Here's how the part is built. I have some questions about the finished solid (model axes, mm). Face numbers are marked on the shaded views. A direction names the side the tool comes from. Round coordinates to 2 decimals unless told otherwise and drop trailing zeros. Loops run counter-clockwise (first coordinate to the right, second up) from the corner with the lowest first, then second, coordinate; pieces in that order, holes last. Notation, with made-up numbers: M 44.25,13 L 73.25,13 A22 cw 73.25,46 Z; hole C 56,0 d3. An arc over 180 degrees is marked long. Answer as CSV lines item,"result".
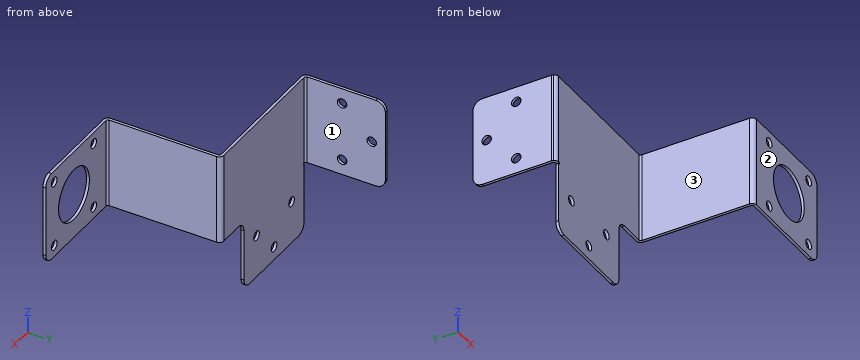
```python
from build123d import *

# Parameters (mm, degrees)
BRIDA_BASE1_DEPTH                = 1.2
BRIDA_START                      = -19
BRIDA_DE_ARISTA1_DEPTH           = 38
BRIDA_START_2                    = -19.6
BRIDA_DE_ARISTA1_2_OUTLINE_W     = 0.5366
BRIDA_DE_ARISTA1_2_OUTLINE_H     = 1.2
BRIDA_DE_ARISTA1_2_DEPTH         = 0.6
BRIDA_DE_ARISTA1_3_DEPTH         = 38
CROQUIS12_R                      = 2
CORTAR_EXTRUIR1_DEPTH            = 1.2
CROQUIS15_R                      = 2
CORTAR_EXTRUIR3_DEPTH            = 1.2
REDONDEO3_R                      = 4
BRIDA_DE_ARISTA2_STRIP_W         = 6.3732
BRIDA_DE_ARISTA2_STRIP_H         = 1.2
BRIDA_DE_ARISTA2_STRIP_CUT_DEPTH = 38
BRIDA_DE_ARISTA2_DEPTH           = 38
BRIDA_DE_ARISTA3_STRIP_W         = 6.3732
BRIDA_DE_ARISTA3_STRIP_H         = 1.2
BRIDA_DE_ARISTA3_STRIP_CUT_DEPTH = 38
BRIDA_DE_ARISTA3_DEPTH           = 38
CROQUIS22_R                      = 2
CROQUIS22_R_2                    = 11
CORTAR_EXTRUIR4_DEPTH            = 1.2
REDONDEO4_R                      = 4


# Read off the part's stored shape, not the designer's step: Brida de arista1
# Sheet-metal steps are written as plain solids
with BuildPart() as part:
    # Croquis1 → Brida base1 (new body)
    with BuildSketch(Plane(origin=(0, 0, 0), x_dir=(1, 0, 0), z_dir=(0, 1, 0))):
        Polygon((-30, -19), (30, -19), (30, 19), (15, 19), (15, 49), (-28, 49), (-28, 19), (-30, 19), align=None)
    extrude(amount=-BRIDA_BASE1_DEPTH)

    # Brida de arista1 outline → Brida de arista1 (cut)
    with BuildSketch(Plane.XY.offset(BRIDA_START)):
        with BuildLine():
            Line((-30, -1.2), (-28.0634, -1.2))
            ThreePointArc((-28.0634, -1.2), (-29.141342484, -0.872269031), (-29.854444388, 0))
            Line((-29.854444388, 0), (-30, 0))
            Line((-30, 0), (-30, -1.2))
        make_face()
    extrude(amount=BRIDA_DE_ARISTA1_DEPTH, mode=Mode.SUBTRACT)

    # Brida de arista1 2 outline → Brida de arista1 2 (cut)
    with BuildSketch(Plane.XY.offset(BRIDA_START_2)):
        with Locations((-27.7317, -0.6)):
            Rectangle(BRIDA_DE_ARISTA1_2_OUTLINE_W, BRIDA_DE_ARISTA1_2_OUTLINE_H)
    extrude(amount=BRIDA_DE_ARISTA1_2_DEPTH, mode=Mode.SUBTRACT)

    # Brida de arista1 3 outline → Brida de arista1 3 (add)
    with BuildSketch(Plane.XY.offset(BRIDA_START)):
        with BuildLine():
            Line((-29.854444388, 0), (-28.0634, 0))
            ThreePointArc((-28.0634, 0), (-28.584254855, 0.215745145), (-28.8, 0.7366))
            Line((-28.8, 0.7366), (-28.8, 33.8))
            Line((-28.8, 33.8), (-30, 33.8))
            Line((-30, 33.8), (-30, 0.7366))
            ThreePointArc((-30, 0.7366), (-29.963262642, 0.361178238), (-29.854444388, 0))
        make_face()
    extrude(amount=BRIDA_DE_ARISTA1_3_DEPTH)

    # Croquis12 → Cortar-Extruir1 (cut)
    with BuildSketch(Plane(origin=(0, 0, 0), x_dir=(1, 0, 0), z_dir=(0, 1, 0))):
        with Locations(Location((6, 30.75, 0), (0, 0, 270))):
            Circle(CROQUIS12_R)
        with Locations(Location((-19, 30.75, 0), (0, 0, 270))):
            Circle(CROQUIS12_R)
        with Locations(Location((-6.5, 43.25, 0), (0, 0, 270))):
            Circle(CROQUIS12_R)
    extrude(amount=-CORTAR_EXTRUIR1_DEPTH, mode=Mode.SUBTRACT)

    # Croquis15 → Cortar-Extruir3 (cut)
    with BuildSketch(Plane.ZY.offset(30)):
        with Locations(Location((-12.5, 15.55, 0), (0, 0, 270))):
            Circle(CROQUIS15_R)
        with Locations(Location((12.5, 15.55, 0), (0, 0, 270))):
            Circle(CROQUIS15_R)
        with Locations(Location((0, 28.05, 0), (0, 0, 270))):
            Circle(CROQUIS15_R)
    extrude(amount=-CORTAR_EXTRUIR3_DEPTH, mode=Mode.SUBTRACT)

    # Redondeo3
    redondeo3_edges = [part.edges().sort_by_distance(p)[0] for p in [
        (-28, -0.6, -49),
        (15, -0.6, -49),
        (15, -0.6, -19),
        (-29.4, 33.8, -19),
        (-29.4, 33.8, 19),
    ]]
    fillet(redondeo3_edges, radius=REDONDEO3_R)

    # Brida de arista2 strip (across the edge) → Brida de arista2 strip cut (cut)
    with BuildSketch(Plane(origin=(30.1, -1.2, -19), x_dir=(-1, 0, 0), z_dir=(0, 0, 1))):
        with Locations((-2.45, -0.6)):
            Rectangle(BRIDA_DE_ARISTA2_STRIP_W, BRIDA_DE_ARISTA2_STRIP_H)
    extrude(amount=BRIDA_DE_ARISTA2_STRIP_CUT_DEPTH, mode=Mode.SUBTRACT)

    # Brida de arista2 section (across the edge) → Brida de arista2 (add)
    with BuildSketch(Plane(origin=(30.1, -1.2, -19), x_dir=(-1, 0, 0), z_dir=(0, 0, 1))):
        with BuildLine():
            Line((-1.2, 0.7366), (-1.2, 46.8))
            Line((-1.2, 46.8), (0, 46.8))
            Line((0, 46.8), (0, 0.7366))
            ThreePointArc((0, 0.7366), (0.215745145, 0.215745145), (0.7366, 0))
            Line((0.7366, 0), (0.7366, -1.2))
            ThreePointArc((0.7366, -1.2), (-0.632782992, -0.632782992), (-1.2, 0.7366))
        make_face()
    extrude(amount=BRIDA_DE_ARISTA2_DEPTH)

    # Brida de arista3 strip (across the edge) → Brida de arista3 strip cut (cut)
    with BuildSketch(Plane(origin=(31.3, -48.1, 19), x_dir=(0, 1, 0), z_dir=(0, 0, -1))):
        with Locations((-2.45, -0.6)):
            Rectangle(BRIDA_DE_ARISTA3_STRIP_W, BRIDA_DE_ARISTA3_STRIP_H)
    extrude(amount=BRIDA_DE_ARISTA3_STRIP_CUT_DEPTH, mode=Mode.SUBTRACT)

    # Brida de arista3 section (across the edge) → Brida de arista3 (add)
    with BuildSketch(Plane(origin=(31.3, -48.1, 19), x_dir=(0, 1, 0), z_dir=(0, 0, -1))):
        with BuildLine():
            Line((-1.2, 0.7366), (-1.2, 43.8))
            Line((-1.2, 43.8), (0, 43.8))
            Line((0, 43.8), (0, 0.7366))
            ThreePointArc((0, 0.7366), (0.215745145, 0.215745145), (0.7366, 0))
            Line((0.7366, 0), (0.7366, -1.2))
            ThreePointArc((0.7366, -1.2), (-0.632782992, -0.632782992), (-1.2, 0.7366))
        make_face()
    extrude(amount=BRIDA_DE_ARISTA3_DEPTH)

    # Croquis22 → Cortar-Extruir4 (cut)
    with BuildSketch(Plane(origin=(0, -48.1, 0), x_dir=(1, 0, 0), z_dir=(0, 1, 0))):
        with Locations(Location((69.1, -14.085, 0), (0, 0, 270))):
            Circle(CROQUIS22_R)
        with Locations(Location((40.93, -14.085, 0), (0, 0, 270))):
            Circle(CROQUIS22_R)
        with Locations(Location((69.1, 14.085, 0), (0, 0, 270))):
            Circle(CROQUIS22_R)
        with Locations(Location((40.93, 14.085, 0), (0, 0, 270))):
            Circle(CROQUIS22_R)
        with Locations(Location((55.015, 0, 0), (0, 0, 270))):
            Circle(CROQUIS22_R_2)
    extrude(amount=-CORTAR_EXTRUIR4_DEPTH, mode=Mode.SUBTRACT)

    # Redondeo4
    redondeo4_edges = [part.edges().sort_by_distance(p)[0] for p in [
        (75.1, -48.7, 19),
        (75.1, -48.7, -19),
    ]]
    fillet(redondeo4_edges, radius=REDONDEO4_R)


solid = part.part
```
1. If I drill on line 1 (Z direction, x = -29.55, y = 15.55); line 2 (X direction, y = -29, z = -11); line 3 (Y direction, x = -29, z = -12), over which ranges is the centre line in solid material (lowest first)? Write a range as [from, to].
Evaluation:
line 1,"z = [-19, -14.5], [-10.5, 10.5], [14.5, 19]"
line 2,"x = [30.1, 31.3]"
line 3,"y = [-0.96, 13.61], [17.49, 33.8]"
2. For P1, Ø12, axis at y = -36, z = 1, coming from the +X side; P2, Ø6, axis at y = -19, z = -10.5, coming from the -X side; P3, Ø4.5, axis at x = -6.5, z = -43.25, coming from the -Y side, each with a flat end and sliding along its axis, tell me the tip position at first contact or that it passes through.
Evaluation:
P1,"stops at x = 31.3"
P2,"stops at x = 30.1"
P3,"stops at y = -1.2"
3. I want a section at A-A, the plane z = 0. Please give me the cut outline in (x, y) (3 decimals).
Evaluation:
outline,"M -30,0.737 A1.937 ccw -28.063,-1.2 L 29.363,-1.2 A0.737 cw 30.1,-1.937 L 30.1,-47.363 A1.937 ccw 32.037,-49.3 L 44.015,-49.3 L 44.015,-48.1 L 32.037,-48.1 A0.737 cw 31.3,-47.363 L 31.3,-1.937 A1.937 ccw 29.363,0 L -28.063,0 A0.737 cw -28.8,0.737 L -28.8,26.05 L -30,26.05 Z; M -30,30.05 L -28.8,30.05 L -28.8,33.8 L -30,33.8 Z; M 66.015,-49.3 L 75.1,-49.3 L 75.1,-48.1 L 66.015,-48.1 Z"
4. I want a section at D-D, the plane x = -19. Please give me the cut outline in (y, z), and give its area (3 significant figures).
Evaluation:
outline,"M -1.2,-49 L 0,-49 L 0,-32.75 L -1.2,-32.75 Z; M -1.2,-28.75 L 0,-28.75 L 0,19 L -1.2,19 Z"
area,"76.8 mm²"
5. I want a section at C-C, the plane y = 16. Please give me the cut outline in (x, z), and give its area (3 significant figures).
Evaluation:
outline,"M -30,-19 L -28.8,-19 L -28.8,-14.45 L -30,-14.45 Z; M -30,-10.55 L -28.8,-10.55 L -28.8,10.55 L -30,10.55 Z; M -30,14.45 L -28.8,14.45 L -28.8,19 L -30,19 Z"
area,"36.2 mm²"
6. I want a section at B-B, the plane x = 69.1. Please give me the cut outline in (y, z) (3 decimals).
Evaluation:
outline,"M -49.3,-19 L -48.1,-19 L -48.1,-16.085 L -49.3,-16.085 Z; M -49.3,-12.085 L -48.1,-12.085 L -48.1,12.085 L -49.3,12.085 Z; M -49.3,16.085 L -48.1,16.085 L -48.1,19 L -49.3,19 Z"
7. Which directions (+Z, -Z, +X, -X, +Y, -Y) give clear straight access to the entire face, cutting with the end or side of a thin tool? Please do the marked faces 1, 2 and 3.
Evaluation:
face 1,"+Z, -Z, +X, +Y"
face 2,"+Z, -Z, +X, -X, -Y"
face 3,"+Z, -Z, -X, -Y"
